Part print with two shaded views. Sizes in mm from the minimum x, y, z corner. Give positions to 0.01 mm unless a question says otherwise; leave off trailing zeros. Order: outer loops, then holes, each group sorted by start corner. A loop starts at its lowest first (then second) coordinate and runs counter-clockwise, first axis right, second up. Notation, with made-up numbers: (12, 77) -> (18, 77) arc R30 cw to (18, 110) -> close; hole circle Ø9 at (2.5, 38.5). An arc over 180 degrees is marked (long way). Answer as CSV lines item,"result".
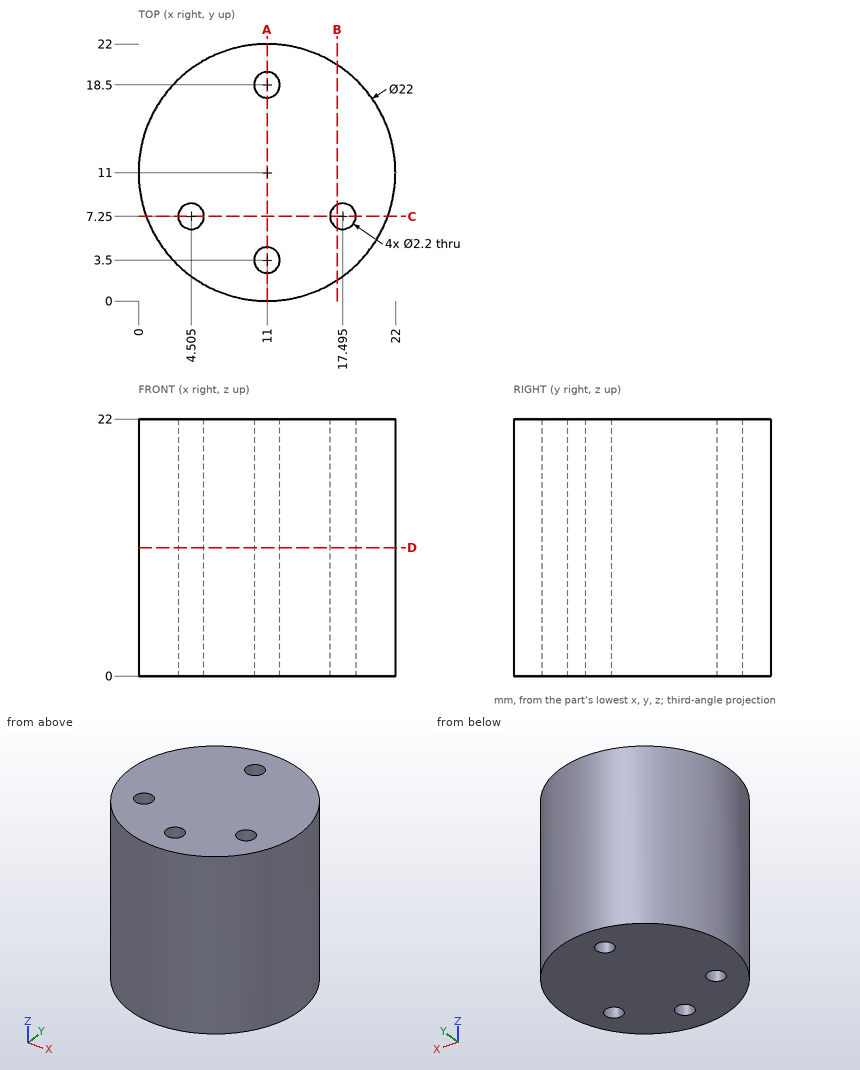
1) Band-saw the part on A-A, the plane x = 11. Write the cut outline in (y, z).
Data:
outline,"(0, 0) -> (2.4, 0) -> (2.4, 22) -> (0, 22) -> close; (4.6, 0) -> (17.4, 0) -> (17.4, 22) -> (4.6, 22) -> close; (19.6, 0) -> (22, 0) -> (22, 22) -> (19.6, 22) -> close"
2) Pin check, flat tips, straight feed: P1, Ø1.5, axis at y = 15, z = 15, coming from the +X side; P2, Ø6, axis at y = 6.5, z = 7.5, coming from the +X side; P3, Ø5, axis at y = 14, z = 16, coming from the -X side. Stop position of each tip, or through.
Data:
P1,"stops at x = 21.51"
P2,"stops at x = 21.9"
P3,"stops at x = 0.01"
3) Band-saw the part on B-B, the plane x = 17. Write the cut outline in (y, z).
Data:
outline,"(1.78, 0) -> (6.27, 0) -> (6.27, 22) -> (1.78, 22) -> close; (8.23, 0) -> (20.22, 0) -> (20.22, 22) -> (8.23, 22) -> close"
4) Band-saw the part on D-D, the plane z = 11. Give the number of separate pieces and of enclosed holes in the cut face, then the cut area to 3 significant figures.
Data:
separate pieces,"1"
enclosed holes,"4"
area,"365 mm2"
5) Wall check: line 1 along Y through (x, z) = (11, 17.25); line 2 along X through (y, z) = (3.75, 13.25); line 3 along X through (y, z) = (3, 10.25). Give the ranges that are in metal, low to high. Write a range as [from, to].
Data:
line 1,"y = [0, 2.4], [4.6, 17.4], [19.6, 22]"
line 2,"x = [2.73, 9.93], [12.07, 19.27]"
line 3,"x = [3.45, 10.02], [11.98, 18.55]"
6) Band-saw the part on C-C, the plane y = 7.25. Write the cut outline in (x, z) (1 decimal), then the cut area to 3 significant figures.
Data:
outline,"(0.7, 0) -> (3.4, 0) -> (3.4, 22) -> (0.7, 22) -> close; (5.6, 0) -> (16.4, 0) -> (16.4, 22) -> (5.6, 22) -> close; (18.6, 0) -> (21.3, 0) -> (21.3, 22) -> (18.6, 22) -> close"
area,"358 mm2"
